Model file for the job. Use its own axes, mm. Round coordinates to 2 decimals unless told otherwise and drop trailing zeros. Loops run counter-clockwise (first coordinate to the right, second up) from the corner with the lowest first, then second, coordinate; pieces in that order, holes last. Notation, with made-up numbers: M 86,-24.5 L 117,-24.5 A26 ccw 117,13.5 Z; hole C -37.75,-15 d5. An arc over 180 degrees is marked long. Use a Markdown table: item, result. Add a question column.
Q1. Pin check, flat tips, straight feed: pin 1 (5 mm diameter, centred on x = 41.5, y = -2, fed in from -Z); pin 2 (3 mm diameter, centred on x = 46.5, y = 1.5, fed in from -Z); pin 3 (6.5 mm diameter, centred on y = 2, z = -90, fed in from +X). Stop position of each tip, or through.
Q2. Probe line 1 (X direction, y = 1.5, z = 0); line 2 (Z direction, x = 19, y = -0.5); line 3 (Z direction, x = 19.5, y = 4.75). List the from-to ranges inside material, lowest first. Write a range as from..to.
Q3. Cut at B-B (z = 0). Give the cut face in (x, y).
Q4. Cut at C-C (z = 35). Give the cut face in (x, y).
Q5. Cut at D-D (x = 21.25). Give the cut face in (y, z), plus the area to 3 significant figures.
Q6. Cut at A-A (x = 48.75). Give the cut face in (y, z), plus the area to 3 significant figures.
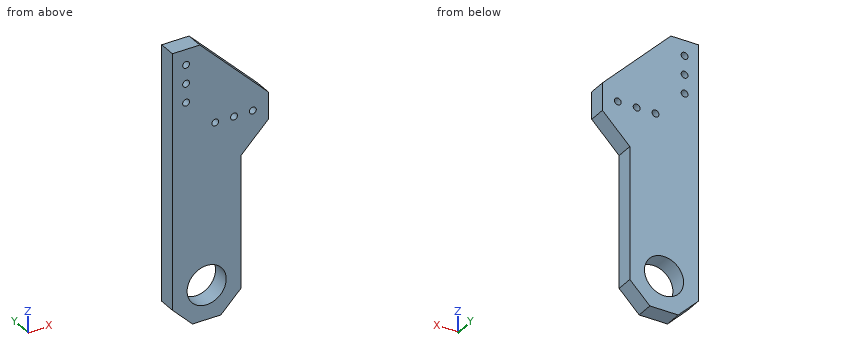
from build123d import *

# Parameters (mm, degrees)
SKETCH1_R           = 14.2875
SKETCH1_R_2         = 2.5
BOSS_EXTRUDE1_DEPTH = 6.35


with BuildPart() as part:
    # Sketch1 → Boss-Extrude1 (new, symmetric)
    with BuildSketch(Plane(origin=(0, 0, 0), x_dir=(1, 0, 0), z_dir=(0, 1, 0))):
        Polygon((-10, -60), (10, -60), (60, -10), (60, 10), (40, 30), (40, 126.725339059), (25.355339059, 141.37), (4.644660941, 141.37), (-10, 126.725339059), align=None)
        with Locations(Location((15, 116.37, 0), (0, 0, 270))):
            Circle(SKETCH1_R, mode=Mode.SUBTRACT)
        with Locations(Location((48.75, 0, 0), (0, 0, 270))):
            Circle(SKETCH1_R_2, mode=Mode.SUBTRACT)
        with Locations(Location((35, 0, 0), (0, 0, 270))):
            Circle(SKETCH1_R_2, mode=Mode.SUBTRACT)
        with Locations(Location((21.25, 0, 0), (0, 0, 270))):
            Circle(SKETCH1_R_2, mode=Mode.SUBTRACT)
        with Locations(Location((0, -48.75, 0), (0, 0, 270))):
            Circle(SKETCH1_R_2, mode=Mode.SUBTRACT)
        with Locations(Location((0, -35, 0), (0, 0, 270))):
            Circle(SKETCH1_R_2, mode=Mode.SUBTRACT)
        with Locations(Location((0, -21.25, 0), (0, 0, 270))):
            Circle(SKETCH1_R_2, mode=Mode.SUBTRACT)
    extrude(amount=BOSS_EXTRUDE1_DEPTH, both=True)


solid = part.part
Checked values:
| question | item | result |
|---|---|---|
| 1 | pin 1 | stops at z = -127.73 |
| 1 | pin 2 | stops at z = -25 |
| 1 | pin 3 | stops at x = 40 |
| 2 | line 1 | x = -10..18.75, 23.75..32.5, 37.5..46.25, 51.25..60 |
| 2 | line 2 | z = -141.37..-130.09, -102.65..-1.09, 1.09..51 |
| 2 | line 3 | z = -141.37..-129.93, -102.81..-1.79, 1.79..50.5 |
| 3 | outline | M -10,-6.35 L 18.75,-6.35 L 18.75,6.35 L -10,6.35 Z; M 23.75,-6.35 L 32.5,-6.35 L 32.5,6.35 L 23.75,6.35 Z; M 37.5,-6.35 L 46.25,-6.35 L 46.25,6.35 L 37.5,6.35 Z; M 51.25,-6.35 L 60,-6.35 L 60,6.35 L 51.25,6.35 Z |
| 4 | outline | M -10,-6.35 L -2.5,-6.35 L -2.5,6.35 L -10,6.35 Z; M 2.5,-6.35 L 35,-6.35 L 35,6.35 L 2.5,6.35 Z |
| 5 | outline | M -6.35,-141.37 L 6.35,-141.37 L 6.35,-129.22 L -6.35,-129.22 Z; M -6.35,-103.52 L 6.35,-103.52 L 6.35,-2.5 L -6.35,-2.5 Z; M -6.35,2.5 L 6.35,2.5 L 6.35,48.75 L -6.35,48.75 Z |
| 5 | area | 2,020 mm^2 |
| 6 | outline | M -6.35,-21.25 L 6.35,-21.25 L 6.35,-2.5 L -6.35,-2.5 Z; M -6.35,2.5 L 6.35,2.5 L 6.35,21.25 L -6.35,21.25 Z |
| 6 | area | 476 mm^2 |
